Check sheet for the drawn part. Datum: minimum x, y, z corner. Units: mm. Round coordinates to 2 decimals unless told otherwise and drop trailing zeros. Write each loop counter-clockwise with the first axis right and the second up, starting at its lowest first coordinate (ties: lowest second). Pieces come first, ordered by that corner, then holes. Notation, with made-up numbers: (7, -32) - (31, -32) arc R22 cw to (31, 1) - close; hole circle Ø5 at (38.5, -27). An arc over 180 degrees is marked (long way). Answer as a JSON object with one key per item and string values.
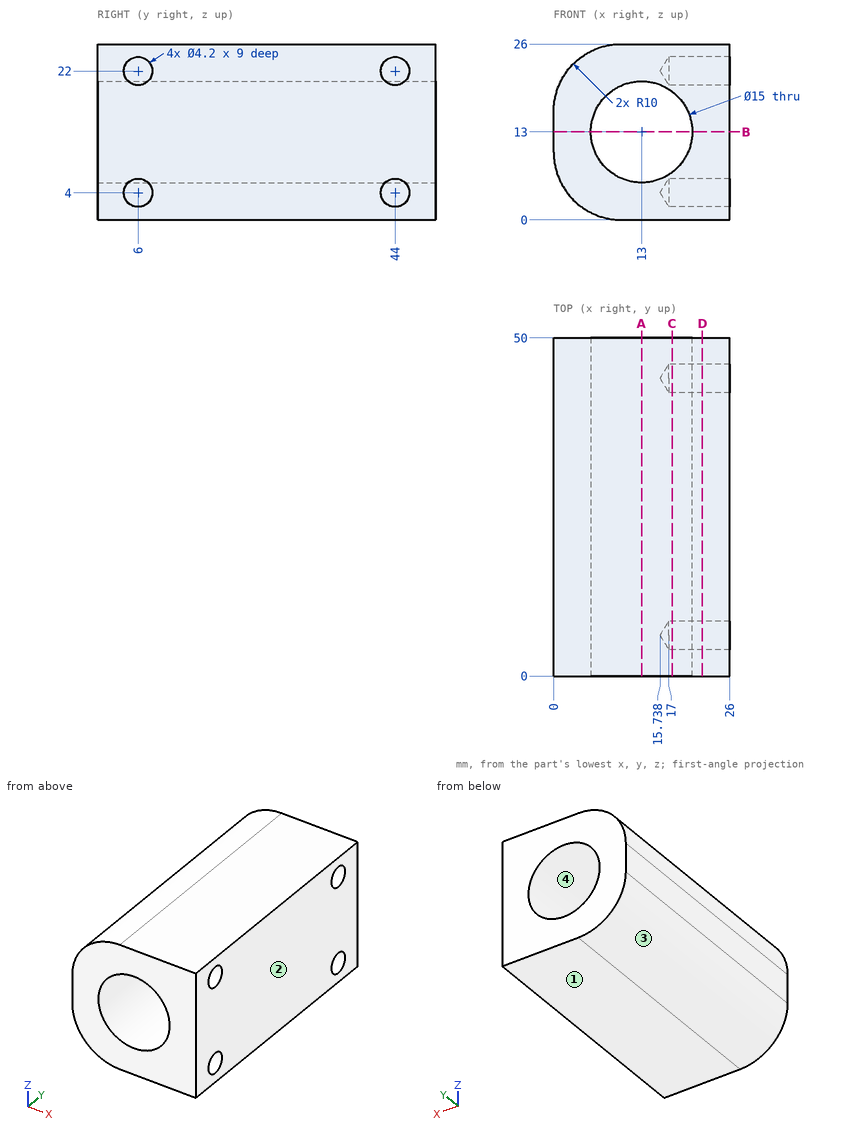
1. Cross-section at D-D (x = 22). Record the boundary of the cut face in (y, z).
Completed:
{"outline": "(0, 0) - (50, 0) - (50, 26) - (0, 26) - close; hole circle Ø4.2 at (6, 4); hole circle Ø4.2 at (6, 22); hole circle Ø4.2 at (44, 4); hole circle Ø4.2 at (44, 22)"}
2. Go/stop test with flat-tipped pins: pin 1 (5.5 mm diameter, centred on y = 6, z = 4, fed in from -X); pin 2 (12 mm diameter, centred on x = 18, z = 15, fed in from +Y); pin 3 (3.5 mm diameter, centred on y = 44, z = 4, fed in from +X); pin 4 (1.5 mm diameter, centred on y = 39.5, z = 4, fed in from -X). Record where each tip stops, or that it passes through.
Completed:
{"pin 1": "stops at x = 0.54", "pin 2": "stops at y = 50", "pin 3": "stops at x = 16.79", "pin 4": "stops at x = 1.49"}
3. Material ranges on probe 1 along Y at (x, z) = (23.5, 4); probe 2 along Z at (x, y) = (21.5, 6); probe 3 along Z at (x, y) = (18, 18), recorded low to high. Write a range as from..to.
Completed:
{"probe 1": "y = 0..3.9, 8.1..41.9, 46.1..50", "probe 2": "z = 0..1.9, 6.1..19.9, 24.1..26", "probe 3": "z = 0..7.41, 18.59..26"}
4. Cross-section at B-B (z = 13). Record the boundary of the cut face in (x, y).
Completed:
{"outline": "(0, 0) - (5.5, 0) - (5.5, 50) - (0, 50) - close; (20.5, 0) - (26, 0) - (26, 50) - (20.5, 50) - close"}
5. Mould release check, pull along X, two halves, no side actions. Record for the marked faces 1, 2, 3 and 4: released by +X, released by -X, zero draft, split by the parting line, or undercut.
Completed:
{"face 1": "zero draft", "face 2": "released by +X", "face 3": "released by -X", "face 4": "undercut"}
6. Cross-section at C-C (x = 17.5). Record the boundary of the cut face in (y, z).
Completed:
{"outline": "(0, 0) - (50, 0) - (50, 7) - (0, 7) - close; (0, 19) - (50, 19) - (50, 26) - (0, 26) - close; hole circle Ø4.2 at (6, 4); hole circle Ø4.2 at (6, 22); hole circle Ø4.2 at (44, 4); hole circle Ø4.2 at (44, 22)"}
7. Cross-section at A-A (x = 13). Record the boundary of the cut face in (y, z).
Completed:
{"outline": "(0, 0) - (50, 0) - (50, 5.5) - (0, 5.5) - close; (0, 20.5) - (50, 20.5) - (50, 26) - (0, 26) - close"}
